Geometry: see drawing. Coordinates: mm, zero at the bounding-box minimum. A direction names the side the tool comes from. Coordinates: 2 decimals unless noted, no trailing zeros. Write each loop counter-clockwise with the first axis right and the second up, starting at its lowest first coordinate (ties: lowest second). Pieces come first, ordered by that corner, then holes. Notation, with made-up numbers: M -38.5,45 L -0.5,45 A28 ccw -0.5,78 Z; hole C 23,3.5 d9. An arc over 180 degrees is marked long. Answer as CSV lines item,"result". Start each with the question number.
1. Contact query for flat-ended pins moving along their axis: pin 1 Ø2 at (y, z) = (129, 4) entering from +X; pin 2 Ø5 at (y, z) = (48, 8) entering from +X (1 decimal); pin 3 Ø6.5 at (x, z) = (8.5, 8) entering from -Y. Output: stop coordinate, or through.
2. Section D-D on x = 16.5. Return the cut outline in (y, z), plus the area to 3 significant figures.
3. Section C-C on y = 179. Return the cut outline in (x, z).
4. Section A-A on y = 6.35. Return the cut outline in (x, z) (1 decimal), plus the area to 3 significant figures.
5. Reachability of the marked faces 4, 5 and 6 from +Z, -Z, +X, -X, +Y, -Y: full face, straight path, thin tool, end or side. Return the list, or none.
6. Mould query, pull axis Y, two halves, no side actions, for the marked faces 1, 2 and 3. Classes: pulls with the +Y half, pulls with the -Y half, needs draft (parallel to the pull), parting line crosses it, or undercut.
7. Line query: probe 1 along Y at (x, z) = (46, 7.25); probe 2 along Y at (x, z) = (34.5, 1) (1 decimal); probe 3 along X at (y, z) = (158, 5.25). Output: solid intervals per line, ascending. Write a range as [from, to].
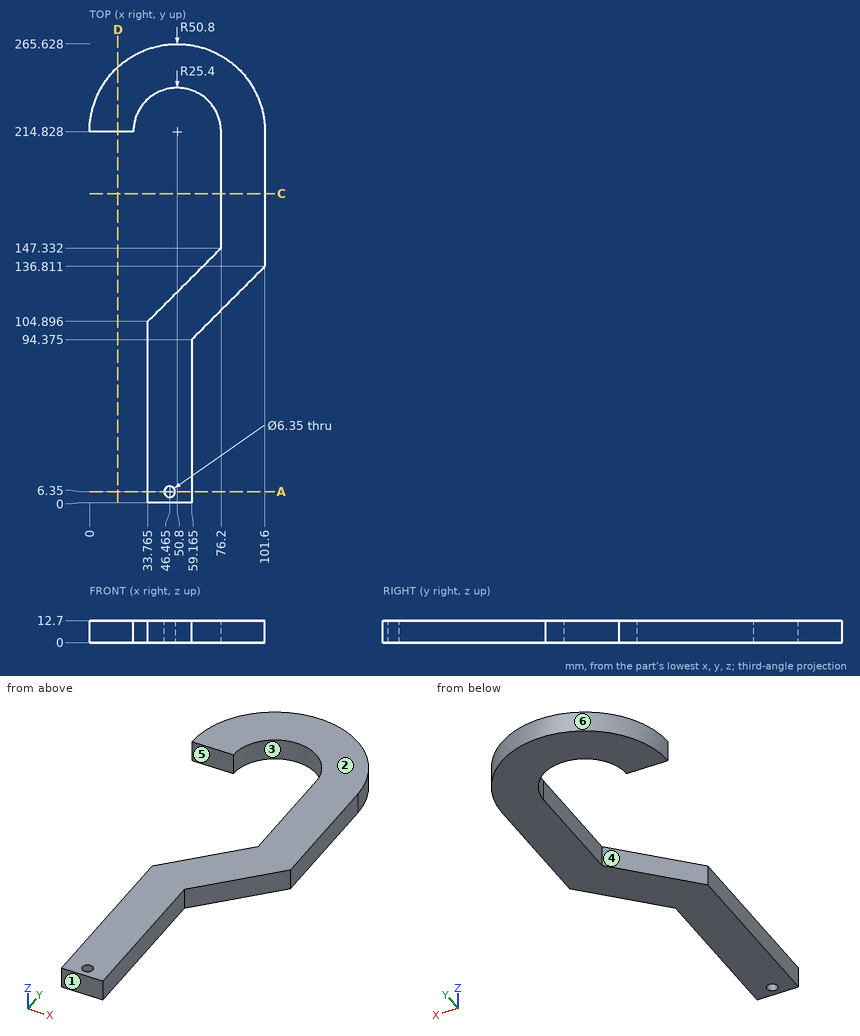
Values:
1,pin 1,"x = 94.79"
1,pin 2,"x = 59.2"
1,pin 3,"y = 214.83"
2,outline,"M 214.83,0 L 252.3,0 L 252.3,12.7 L 214.83,12.7 Z"
2,area,"476 mm²"
3,outline,"M 76.2,0 L 101.6,0 L 101.6,12.7 L 76.2,12.7 Z"
4,outline,"M 33.8,0 L 43.3,0 L 43.3,12.7 L 33.8,12.7 Z; M 49.6,0 L 59.2,0 L 59.2,12.7 L 49.6,12.7 Z"
4,area,"242 mm²"
5,face 4,"+Z, -Z, -X"
5,face 5,"+Z, -Z, -X, -Y"
5,face 6,"+Z, -Z, +Y"
6,face 1,"pulls with the -Y half"
6,face 2,"needs draft"
6,face 3,"undercut"
7,probe 1,"[0, 3.21], [9.49, 117.13], [239.77, 265.4]"
7,probe 2,"[0, 105.6], [234.3, 262.9]"
7,probe 3,"[76.2, 101.6]"
